```python
from build123d import *


with BuildPart() as part:
    # 草图1 → 旋转1 (revolve)
    with BuildSketch(Plane.XY, mode=Mode.PRIVATE) as revolve_1_sk:
        Polygon((23.8, -0.545464411), (23.8, 7.954535589), (28, 7.954535589), (28, 2.954535589), (25.4, 2.954535589), (25.4, 1.954535589), (26, 1.954535589), (26, -0.545464411), align=None)
    revolve(revolve_1_sk.sketch.rotate(Axis((0, 16.886018237, 0), (0, -1, 0)), 180), axis=Axis((0, 16.886018237, 0), (0, -1, 0)))  # turned: the seam where the file's is


solid = part.part
```
The model under review builds one solid part; all positions refer to its coordinate system, in mm. A direction names the side the tool comes from. Coordinates: 2 decimals unless noted, no trailing zeros. Write each loop counter-clockwise with the first axis right and the second up, starting at its lowest first coordinate (ties: lowest second). Pieces come first, ordered by that corner, then holes.
1) Machinability: for faces 4 (the face through (20.633, 0.687, 15.821)), 5 (the face through (-6, 2.955, 25)), 6 (the face through (17.542, 3.764, -16.085)), which of the approach directions +Z, -Z, +X, -X, +Y, -Y give a long, thin tool a straight path to every point of the face, cutting with its end or side? Answer none if there is none.
2) Clearance check with flat-ended pins moving along their axes: pin 1 Ø17 at (x, z) = (-8.5, -11) entering from -Y; pin 2 Ø5 at (x, y) = (-20.5, 4) entering from -Z; pin 3 Ø5 at (x, y) = (-7.5, 3) entering from -Z; pin 4 Ø1.5 at (x, y) = (21.5, 3.5) entering from -Z. State where each tip first meets the part, or that it passes through.
3) To check wall thickness, follow probe 1 along Z at (x, y) = (0, 2.75); probe 2 along Z at (x, y) = (0, 4); probe 3 along X at (y, z) = (4.25, 18). State the ranges of each line that lie inside material, in increasing order.
4) We need section B-B on z = 0. State the section outline as (x, y) points.
5) We need section A-A on x = 0. State the section outline as (y, z) points.
6) The part is to be moulded in two halves that separate along Y. For faces 1 (the face through (-25.865, 5.42, 10.724)), 2 (the face through (-11.721, 2.448, 22.534)), 3 (the face through (-11.4, -0.545, 21.1)), say which applies: pulls with the +Y half, pulls with the -Y half, needs draft (parallel to the pull), parting line crosses it, or undercut.
Answer list:
1. face 4: -Y
1. face 5: none
1. face 6: +Y, -Y
2. pin 1: passes through
2. pin 2: stops at z = -21.45
2. pin 3: stops at z = -27.55
2. pin 4: stops at z = -18.8
3. probe 1: z = -25.4 to -23.8, 23.8 to 25.4
3. probe 2: z = -28 to -23.8, 23.8 to 28
3. probe 3: x = -21.45 to -15.57, 15.57 to 21.45
4. outline: (-28, 2.95) - (-25.4, 2.95) - (-25.4, 1.95) - (-26, 1.95) - (-26, -0.55) - (-23.8, -0.55) - (-23.8, 7.95) - (-28, 7.95) - close; (23.8, -0.55) - (26, -0.55) - (26, 1.95) - (25.4, 1.95) - (25.4, 2.95) - (28, 2.95) - (28, 7.95) - (23.8, 7.95) - close
5. outline: (-0.55, -26) - (1.95, -26) - (1.95, -25.4) - (2.95, -25.4) - (2.95, -28) - (7.95, -28) - (7.95, -23.8) - (-0.55, -23.8) - close; (-0.55, 23.8) - (7.95, 23.8) - (7.95, 28) - (2.95, 28) - (2.95, 25.4) - (1.95, 25.4) - (1.95, 26) - (-0.55, 26) - close
6. face 1: needs draft
6. face 2: undercut
6. face 3: pulls with the -Y half
